Part model, mm, in its own coordinate system. A direction names the side the tool comes from. Give positions to 0.01 mm unless a question says otherwise; leave off trailing zeros. Write each loop counter-clockwise with the first axis right and the second up, starting at its lowest first coordinate (ties: lowest second). Pieces come first, ordered by that corner, then holes. Notation, with made-up numbers: M -36.5,24.25 L 20.5,24.25 A30 ccw 20.5,46.25 Z; hole C 34.5,-3.75 d5. An arc over 180 degrees is marked long. Use a Markdown table: item, result. Add a question column.
from build123d import *

# Parameters (mm, degrees)
SKETCH1_W           = 21
SKETCH1_H           = 19
SKETCH1_R           = 1.5
BOSS_EXTRUDE1_DEPTH = 19
CHAMFER1_SIZE       = 1.5
SKETCH2_W           = 27
SKETCH2_H           = 27
BOSS_EXTRUDE2_DEPTH = 8
FILLET1_R           = 10
CHAMFER2_SIZE       = 0.8


with BuildPart() as part:
    # Sketch1 → Boss-Extrude1 (new body)
    with BuildSketch(Plane(origin=(0, 0, 0), x_dir=(1, 0, 0), z_dir=(0, 1, 0))):
        with Locations((10.5, 9.5)):
            Rectangle(SKETCH1_W, SKETCH1_H)
        with Locations(Location((12, 13.5, 0), (0, 0, 270))):
            Circle(SKETCH1_R, mode=Mode.SUBTRACT)
        with Locations(Location((12, 5.5, 0), (0, 0, 270))):
            Circle(SKETCH1_R, mode=Mode.SUBTRACT)
    extrude(amount=BOSS_EXTRUDE1_DEPTH)

    # Chamfer1
    chamfer1_edges = [part.edges().sort_by_distance(p)[0] for p in [
        (0, 19, -9.5),
        (0, 0, -9.5),
        (0, 9.5, -19),
        (0, 9.5, 0),
    ]]
    chamfer(chamfer1_edges, length=CHAMFER1_SIZE)

    # Sketch2 → Boss-Extrude2 (add)
    with BuildSketch(Plane(origin=(21, 0, 0), x_dir=(0, 0, -1), z_dir=(1, 0, 0))):
        with Locations((9.5, 9.5)):
            Rectangle(SKETCH2_W, SKETCH2_H)
    extrude(amount=BOSS_EXTRUDE2_DEPTH)

    # Fillet1
    # the kernel refuses this fillet: 10 mm, written as the material it adds along each edge
    with BuildSketch(Plane(origin=(21, 19, 0), x_dir=(0, 1, 0), z_dir=(0, 0, -1))) as fillet1_piece_1_section:
        with BuildLine():
            CenterArc((10, -8), FILLET1_R, 126.869897646, 53.130102354)
            Line((0, -8), (-0.2, -8))
            Line((-0.2, -8), (-0.2, 0))
            Line((-0.2, 0), (0, 0.2))
            ThreePointArc((0, 0.2), (2, 0.2), (3.88, 0.16))
            Line((3.88, 0.16), (4, 0))
        make_face()
    fillet1_piece_1 = extrude(amount=19, mode=Mode.PRIVATE)
    fillet1_piece_1 = fillet1_piece_1 - Plane(origin=(12, 20.025432283, -13.5), x_dir=(0, 0, 1), z_dir=(0, -1, 0)) * Cylinder(1.5, 70, mode=Mode.PRIVATE)
    fillet1_piece_1 = fillet1_piece_1 - Plane(origin=(12, 20.025432283, -5.5), x_dir=(0, 0, 1), z_dir=(0, -1, 0)) * Cylinder(1.5, 70, mode=Mode.PRIVATE)
    add(fillet1_piece_1)
    with BuildSketch(Plane(origin=(21, 0, 0), x_dir=(0, -1, 0), z_dir=(0, 0, -1))) as fillet1_piece_2_section:
        with BuildLine():
            CenterArc((10, 8), FILLET1_R, 180, 53.130102354)
            Line((0, 8), (-0.2, 8))
            Line((-0.2, 8), (-0.2, 0))
            Line((-0.2, 0), (0, -0.2))
            ThreePointArc((0, -0.2), (2, -0.2), (3.88, -0.16))
            Line((3.88, -0.16), (4, 0))
        make_face()
    fillet1_piece_2 = extrude(amount=19, mode=Mode.PRIVATE)
    fillet1_piece_2 = fillet1_piece_2 - Plane(origin=(12, -1.025432283, -13.5), x_dir=(0, 0, 1), z_dir=(0, -1, 0)) * Cylinder(1.5, 70, mode=Mode.PRIVATE)
    fillet1_piece_2 = fillet1_piece_2 - Plane(origin=(12, -1.025432283, -5.5), x_dir=(0, 0, 1), z_dir=(0, -1, 0)) * Cylinder(1.5, 70, mode=Mode.PRIVATE)
    add(fillet1_piece_2)
    with BuildSketch(Plane(origin=(21, 0, -19), x_dir=(0, 0, -1), z_dir=(0, 1, 0))) as fillet1_piece_3:
        with BuildLine():
            CenterArc((10, 8), FILLET1_R, 180, 53.130102354)
            Line((0, 8), (-0.2, 8))
            Line((-0.2, 8), (-0.2, 0))
            Line((-0.2, 0), (0, -0.2))
            ThreePointArc((0, -0.2), (2, -0.2), (3.88, -0.16))
            Line((3.88, -0.16), (4, 0))
        make_face()
    extrude(amount=19)
    with BuildSketch(Plane(origin=(21, 0, 0), x_dir=(0, 0, 1), z_dir=(0, 1, 0))) as fillet1_piece_4:
        with BuildLine():
            CenterArc((10, -8), FILLET1_R, 126.869897646, 53.130102354)
            Line((0, -8), (-0.2, -8))
            Line((-0.2, -8), (-0.2, 0))
            Line((-0.2, 0), (0, 0.2))
            ThreePointArc((0, 0.2), (2, 0.2), (3.88, 0.16))
            Line((3.88, 0.16), (4, 0))
        make_face()
    extrude(amount=19)
    with BuildSketch(Plane(origin=(21, 19, 20), x_dir=(0, 1, 0), z_dir=(0, 0, -1))) as fillet1_piece_5a_section:
        with BuildLine():
            CenterArc((10, -8), FILLET1_R, 126.869897646, 53.130102354)
            Line((0, -8), (-0.2, -8))
            Line((-0.2, -8), (-0.2, 0))
            Line((-0.2, 0), (0, 0.2))
            ThreePointArc((0, 0.2), (2, 0.2), (3.88, 0.16))
            Line((3.88, 0.16), (4, 0))
        make_face()
    fillet1_piece_5a = extrude(amount=39, mode=Mode.PRIVATE)
    fillet1_piece_5a = split(fillet1_piece_5a, bisect_by=Plane(origin=(18.941165886, 20.023885124, 4), z_dir=(0, 0, -1)), keep=Keep.TOP, mode=Mode.PRIVATE)
    fillet1_piece_5a = split(fillet1_piece_5a, bisect_by=Plane(origin=(18.941165886, 20.023885124, 0), z_dir=(0, 0, 1)), keep=Keep.TOP, mode=Mode.PRIVATE)
    with BuildSketch(Plane(origin=(21, 0, 0), x_dir=(0, 0, 1), z_dir=(0, 1, 0))) as fillet1_piece_5b_section:
        with BuildLine():
            CenterArc((10, -8), FILLET1_R, 126.869897646, 53.130102354)
            Line((0, -8), (-0.2, -8))
            Line((-0.2, -8), (-0.2, 0))
            Line((-0.2, 0), (0, 0.2))
            ThreePointArc((0, 0.2), (2, 0.2), (3.88, 0.16))
            Line((3.88, 0.16), (4, 0))
        make_face()
    fillet1_piece_5b = extrude(amount=39, mode=Mode.PRIVATE)
    fillet1_piece_5b = split(fillet1_piece_5b, bisect_by=Plane(origin=(18.941165886, 23, 1.023885124), z_dir=(0, -1, 0)), keep=Keep.TOP, mode=Mode.PRIVATE)
    fillet1_piece_5b = split(fillet1_piece_5b, bisect_by=Plane(origin=(18.941165886, 19, 1.023885124), z_dir=(0, 1, 0)), keep=Keep.TOP, mode=Mode.PRIVATE)
    fillet1_piece_5 = fillet1_piece_5a & fillet1_piece_5b
    add(fillet1_piece_5)
    with BuildSketch(Plane(origin=(21, 0, -19), x_dir=(0, 0, -1), z_dir=(0, 1, 0))) as fillet1_piece_6a_section:
        with BuildLine():
            CenterArc((10, 8), FILLET1_R, 180, 53.130102354)
            Line((0, 8), (-0.2, 8))
            Line((-0.2, 8), (-0.2, 0))
            Line((-0.2, 0), (0, -0.2))
            ThreePointArc((0, -0.2), (2, -0.2), (3.88, -0.16))
            Line((3.88, -0.16), (4, 0))
        make_face()
    fillet1_piece_6a = extrude(amount=39, mode=Mode.PRIVATE)
    fillet1_piece_6a = split(fillet1_piece_6a, bisect_by=Plane(origin=(18.941165886, 23, -20.023885124), z_dir=(0, -1, 0)), keep=Keep.TOP, mode=Mode.PRIVATE)
    fillet1_piece_6a = split(fillet1_piece_6a, bisect_by=Plane(origin=(18.941165886, 19, -20.023885124), z_dir=(0, 1, 0)), keep=Keep.TOP, mode=Mode.PRIVATE)
    with BuildSketch(Plane(origin=(21, 19, 0), x_dir=(0, 1, 0), z_dir=(0, 0, -1))) as fillet1_piece_6b_section:
        with BuildLine():
            CenterArc((10, -8), FILLET1_R, 126.869897646, 53.130102354)
            Line((0, -8), (-0.2, -8))
            Line((-0.2, -8), (-0.2, 0))
            Line((-0.2, 0), (0, 0.2))
            ThreePointArc((0, 0.2), (2, 0.2), (3.88, 0.16))
            Line((3.88, 0.16), (4, 0))
        make_face()
    fillet1_piece_6b = extrude(amount=39, mode=Mode.PRIVATE)
    fillet1_piece_6b = split(fillet1_piece_6b, bisect_by=Plane(origin=(18.941165886, 20.023885124, -23), z_dir=(0, 0, 1)), keep=Keep.TOP, mode=Mode.PRIVATE)
    fillet1_piece_6b = split(fillet1_piece_6b, bisect_by=Plane(origin=(18.941165886, 20.023885124, -19), z_dir=(0, 0, -1)), keep=Keep.TOP, mode=Mode.PRIVATE)
    fillet1_piece_6 = fillet1_piece_6a & fillet1_piece_6b
    add(fillet1_piece_6)
    with BuildSketch(Plane(origin=(21, 0, 20), x_dir=(0, -1, 0), z_dir=(0, 0, -1))) as fillet1_piece_7a_section:
        with BuildLine():
            CenterArc((10, 8), FILLET1_R, 180, 53.130102354)
            Line((0, 8), (-0.2, 8))
            Line((-0.2, 8), (-0.2, 0))
            Line((-0.2, 0), (0, -0.2))
            ThreePointArc((0, -0.2), (2, -0.2), (3.88, -0.16))
            Line((3.88, -0.16), (4, 0))
        make_face()
    fillet1_piece_7a = extrude(amount=39, mode=Mode.PRIVATE)
    fillet1_piece_7a = split(fillet1_piece_7a, bisect_by=Plane(origin=(18.941165886, -1.023885124, 4), z_dir=(0, 0, -1)), keep=Keep.TOP, mode=Mode.PRIVATE)
    fillet1_piece_7a = split(fillet1_piece_7a, bisect_by=Plane(origin=(18.941165886, -1.023885124, 0), z_dir=(0, 0, 1)), keep=Keep.TOP, mode=Mode.PRIVATE)
    with BuildSketch(Plane(origin=(21, -20, 0), x_dir=(0, 0, 1), z_dir=(0, 1, 0))) as fillet1_piece_7b_section:
        with BuildLine():
            CenterArc((10, -8), FILLET1_R, 126.869897646, 53.130102354)
            Line((0, -8), (-0.2, -8))
            Line((-0.2, -8), (-0.2, 0))
            Line((-0.2, 0), (0, 0.2))
            ThreePointArc((0, 0.2), (2, 0.2), (3.88, 0.16))
            Line((3.88, 0.16), (4, 0))
        make_face()
    fillet1_piece_7b = extrude(amount=39, mode=Mode.PRIVATE)
    fillet1_piece_7b = split(fillet1_piece_7b, bisect_by=Plane(origin=(18.941165886, -4, 1.023885124), z_dir=(0, 1, 0)), keep=Keep.TOP, mode=Mode.PRIVATE)
    fillet1_piece_7b = split(fillet1_piece_7b, bisect_by=Plane(origin=(18.941165886, 0, 1.023885124), z_dir=(0, -1, 0)), keep=Keep.TOP, mode=Mode.PRIVATE)
    fillet1_piece_7 = fillet1_piece_7a & fillet1_piece_7b
    add(fillet1_piece_7)
    with BuildSketch(Plane(origin=(21, 0, 0), x_dir=(0, -1, 0), z_dir=(0, 0, -1))) as fillet1_piece_8a_section:
        with BuildLine():
            CenterArc((10, 8), FILLET1_R, 180, 53.130102354)
            Line((0, 8), (-0.2, 8))
            Line((-0.2, 8), (-0.2, 0))
            Line((-0.2, 0), (0, -0.2))
            ThreePointArc((0, -0.2), (2, -0.2), (3.88, -0.16))
            Line((3.88, -0.16), (4, 0))
        make_face()
    fillet1_piece_8a = extrude(amount=39, mode=Mode.PRIVATE)
    fillet1_piece_8a = split(fillet1_piece_8a, bisect_by=Plane(origin=(18.941165886, -1.023885124, -23), z_dir=(0, 0, 1)), keep=Keep.TOP, mode=Mode.PRIVATE)
    fillet1_piece_8a = split(fillet1_piece_8a, bisect_by=Plane(origin=(18.941165886, -1.023885124, -19), z_dir=(0, 0, -1)), keep=Keep.TOP, mode=Mode.PRIVATE)
    with BuildSketch(Plane(origin=(21, -20, -19), x_dir=(0, 0, -1), z_dir=(0, 1, 0))) as fillet1_piece_8b_section:
        with BuildLine():
            CenterArc((10, 8), FILLET1_R, 180, 53.130102354)
            Line((0, 8), (-0.2, 8))
            Line((-0.2, 8), (-0.2, 0))
            Line((-0.2, 0), (0, -0.2))
            ThreePointArc((0, -0.2), (2, -0.2), (3.88, -0.16))
            Line((3.88, -0.16), (4, 0))
        make_face()
    fillet1_piece_8b = extrude(amount=39, mode=Mode.PRIVATE)
    fillet1_piece_8b = split(fillet1_piece_8b, bisect_by=Plane(origin=(18.941165886, -4, -20.023885124), z_dir=(0, 1, 0)), keep=Keep.TOP, mode=Mode.PRIVATE)
    fillet1_piece_8b = split(fillet1_piece_8b, bisect_by=Plane(origin=(18.941165886, 0, -20.023885124), z_dir=(0, -1, 0)), keep=Keep.TOP, mode=Mode.PRIVATE)
    fillet1_piece_8 = fillet1_piece_8a & fillet1_piece_8b
    add(fillet1_piece_8)

    # Chamfer2
    chamfer2_edges = [part.edges().sort_by_distance(p)[0] for p in [
        (29, 9.5, 4),
        (29, -4, -9.5),
        (29, 9.5, -23),
        (29, 23, -9.5),
    ]]
    chamfer(chamfer2_edges, length=CHAMFER2_SIZE)


solid = part.part
1. Tool access for faces 5 (the flat face through (7, 19, -10)), 6 (the flat face through (7, 9, -19)), 7 (the flat face through (0.8, 9.4, -0.7)): list every direction of +Z, -Z, +X, -X, +Y, -Y with a clear straight run to the whole face (end or side of a thin tool).
2. Cut at A-A (z = -5.5). Write the cut outline in (x, y), then the cut area to 3 significant figures.
3. Cut at D-D (y = 7.5). Write the cut outline in (x, z).
4. Drill centre lines: probe 1 along Z at (x, y) = (12, 15.25); probe 2 along X at (y, z) = (10.5, -5.5); probe 3 along Z at (x, y) = (5, 16.75). Where is each one in solid material? Low to high. Write a range as [from, to].
5. Cut at C-C (z = -9.5). Write the cut outline in (x, y), then the cut area to 3 significant figures.
6. Flat gauge pins, fed straight in: pin 1 (9 mm diameter, centred on x = 8.5, y = 12.5, fed in from +Z); pin 2 (1.5 mm diameter, centred on x = 16, z = -19, fed in from +Y); pin 3 (5 mm diameter, centred on x = 20.5, z = -5.5, fed in from +Y); pin 4 (2 mm diameter, centred on x = 7, y = 2.5, fed in from -Z). Where does each tip first touch, or does it go through?
7. Cut at B-B (x = 12). Write the cut outline in (y, z).
8. Mould opens along X. For faces 1 (the flat face through (7, 9, 0)), 2 (the flat face through (28.6, 9.3, 3.6)), 3 (the flat face through (0, 9, -9)), 4 (the cylindrical face through (12.9, 9.4, -6.7)) say: released by +X, released by -X, zero draft, split by the parting line, or undercut.
A:
| question | item | result |
|---|---|---|
| 1 | face 5 | +Z, -Z, -X, +Y |
| 1 | face 6 | -Z, -X, +Y, -Y |
| 1 | face 7 | +Z, -X, +Y, -Y |
| 2 | outline | M 0,1.5 L 1.5,0 L 10.5,0 L 10.5,19 L 1.5,19 L 0,17.5 Z; M 13.5,-0.01 A10 cw 21,-4 L 28.2,-4 L 29,-3.2 L 29,22.2 L 28.2,23 L 21,23 A10 cw 13.5,19.01 Z |
| 2 | area | 574 mm² |
| 3 | outline | M 0,-17.5 L 1.5,-19 L 13,-19 A10 cw 21,-23 L 28.2,-23 L 29,-22.2 L 29,3.2 L 28.2,4 L 21,4 A10 cw 13,0 L 1.5,0 L 0,-1.5 Z; hole C 12,-13.5 d3; hole C 12,-5.5 d3 |
| 4 | probe 1 | z = [-19, -15], [-12, -7], [-4, 0] |
| 4 | probe 2 | x = [0, 10.5], [13.5, 29] |
| 4 | probe 3 | z = [-19, 0] |
| 5 | outline | M 0,1.5 L 1.5,0 L 13,0 A10 cw 21,-4 L 28.2,-4 L 29,-3.2 L 29,22.2 L 28.2,23 L 21,23 A10 cw 13,19 L 1.5,19 L 0,17.5 Z |
| 5 | area | 631 mm² |
| 6 | pin 1 | stops at z = 0 |
| 6 | pin 2 | stops at y = 19.73 |
| 6 | pin 3 | stops at y = 23 |
| 6 | pin 4 | stops at z = -19 |
| 7 | outline | M 0,-19 L 19,-19 L 19,-15 L 0,-15 Z; M 0,-12 L 19,-12 L 19,-7 L 0,-7 Z; M 0,-4 L 19,-4 L 19,0 L 0,0 Z |
| 8 | face 1 | zero draft |
| 8 | face 2 | released by +X |
| 8 | face 3 | released by -X |
| 8 | face 4 | undercut |
